Build history of the part. All positions in model axes, mm. Coordinates: 2 decimals unless noted, no trailing zeros. Write each loop counter-clockwise with the first axis right and the second up, starting at its lowest first coordinate (ties: lowest second). Pieces come first, ordered by that corner, then holes. Notation, with made-up numbers: M 52.25,48.25 L 61.25,48.25 A4 cw 61.25,53.25 Z; hole C 70.5,-11 d11. An arc over 180 degrees is marked long. Use CSV: the item, a comma, the result in double quotes. Start each with the question number.
```python
from build123d import *

# Parameters (mm, degrees)
SKETCH_1_W      = 20
SKETCH_1_H      = 40
SKETCH_1_R      = 1.65
EXTRUDE_1_DEPTH = 10
FILLET_1_R      = 2


with BuildPart() as part:
    # 草图1 → 凸台-拉伸1 (new body)
    with BuildSketch(Plane.XY):
        Rectangle(SKETCH_1_W, SKETCH_1_H)
        with Locations((0, 15)):
            Circle(SKETCH_1_R, mode=Mode.SUBTRACT)
        with Locations(Location((0, -15, 0), (0, 0, 180))):
            Circle(SKETCH_1_R, mode=Mode.SUBTRACT)
    extrude(amount=EXTRUDE_1_DEPTH)

    # 圆角1
    fillet_1_edges = [part.edges().sort_by_distance(p)[0] for p in [
        (10, -20, 5),
        (-10, -20, 5),
        (-10, 20, 5),
        (10, 20, 5),
    ]]
    fillet(fillet_1_edges, radius=FILLET_1_R)


solid = part.part
```
1. Slice it at C-C (y = 15). List the corners of the cut face in (x, z), and give its area (3 significant figures).
2. Drill centre lines: line 1 along Y through (x, z) = (0, 7); line 2 along X through (y, z) = (-15, 5.5); line 3 along Y through (x, z) = (-1, 7.25). Where is each one in solid material? Low to high. Write a range as from..to.
3. Flat gauge pin, fed straight in: pin 1 (4 mm diameter, centred on x = 0, y = -15, fed in from +Z). Where does the tip first touch, or does it go through?
4. Slice it at B-B (z = 2). List the corners of the cut face in (x, y), and give its area (3 significant figures).
5. Pull direction X, two halves, no side cores. Call faces 1 (the flat face through (0, 0, 0)), 2 (the cylindrical face through (-0.89, -16.39, 4.93)), 3 (the flat face through (10, 0, 5)): pulls with the +X half, pulls with the -X half, needs draft (parallel to the pull), parting line crosses it, or undercut.
6. Slice it at A-A (x = 0). List the corners of the cut face in (y, z), and give its area (3 significant figures).
Established:
1,outline,"M -10,0 L -1.65,0 L -1.65,10 L -10,10 Z; M 1.65,0 L 10,0 L 10,10 L 1.65,10 Z"
1,area,"167 mm2"
2,line 1,"y = -20..-16.65, -13.35..13.35, 16.65..20"
2,line 2,"x = -10..-1.65, 1.65..10"
2,line 3,"y = -20..-16.31, -13.69..13.69, 16.31..20"
3,pin 1,"stops at z = 10"
4,outline,"M -10,-18 A2 ccw -8,-20 L 8,-20 A2 ccw 10,-18 L 10,18 A2 ccw 8,20 L -8,20 A2 ccw -10,18 Z; hole C 0,-15 d3.3; hole C 0,15 d3.3"
4,area,"779 mm2"
5,face 1,"needs draft"
5,face 2,"undercut"
5,face 3,"pulls with the +X half"
6,outline,"M -20,0 L -16.65,0 L -16.65,10 L -20,10 Z; M -13.35,0 L 13.35,0 L 13.35,10 L -13.35,10 Z; M 16.65,0 L 20,0 L 20,10 L 16.65,10 Z"
6,area,"334 mm2"
